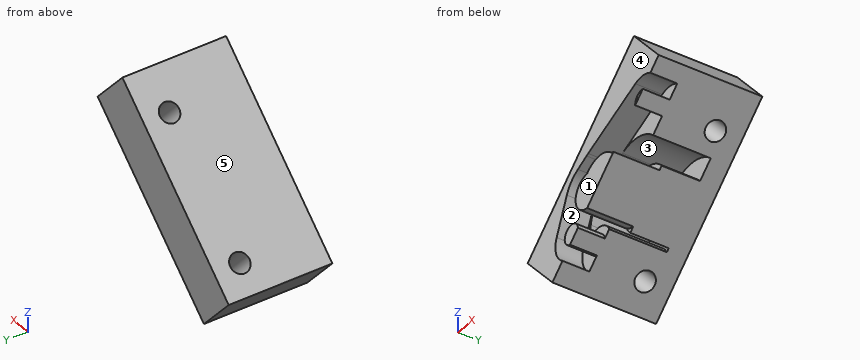
```python
from build123d import *
from build123d.topology import SkipClean

# Parameters (mm, degrees)
SKETCH2_R           = 2.5
BOSS_EXTRUDE1_DEPTH = 7
FILLET1_R           = 90
BOSS_EXTRUDE3_DEPTH = 15
SKETCH4_R           = 8
CUT_EXTRUDE1_DEPTH  = 10
BOSS_EXTRUDE4_START = 10
BOSS_EXTRUDE4_DEPTH = 10
BOSS_EXTRUDE5_DEPTH = 27
SKETCH7_R           = 2.5
CUT_EXTRUDE2_DEPTH  = 37
INTERSECT3_DEPTH    = 27


with BuildPart() as part:
    # Sketch2 → Boss-Extrude1 (new body)
    with BuildSketch(Plane(origin=(0, 0, 0), x_dir=(1, 0, 0), z_dir=(0, 1, 0))):
        with BuildLine():
            Line((-4.24846021, -9.602113613), (13.572308451, -17.486922065))
            ThreePointArc((13.572308451, -17.486922065), (20.638500285, -15.805826469), (20.907079545, -8.547382103))
            Line((20.907079545, -8.547382103), (11.451696022, 4.891208687))
            ThreePointArc((11.451696022, 4.891208687), (9.270724445, 7.034926316), (6.472222222, 8.268031175))
            ThreePointArc((6.472222222, 8.268031175), (4.86754966, 9.30359932), (3.101845071, 10.031378627))
            Line((3.101845071, 10.031378627), (-8.821699821, 13.718308443))
            ThreePointArc((-8.821699821, 13.718308443), (-15.091857172, 11.987583677), (-16.147811194, 5.569231667))
            Line((-16.147811194, 5.569231667), (-12.308520784, -3.358124948))
            ThreePointArc((-12.308520784, -3.358124948), (-9.971976629, -6.504419403), (-6.472222222, -8.268031175))
            ThreePointArc((-6.472222222, -8.268031175), (-5.401685102, -9.003987898), (-4.24846021, -9.602113613))
        make_face()
        with Locations(Location((16, -12, 0), (0, 0, 270))):
            Circle(SKETCH2_R, mode=Mode.SUBTRACT)
        with Locations(Location((-10.604337088, 7.953252816, 0), (0, 0, 270))):
            Circle(SKETCH2_R, mode=Mode.SUBTRACT)
        with BuildLine():
            ThreePointArc((-4.694444444, -4.495797077), (0, -6.5), (4.694444444, -4.495797077))
            ThreePointArc((4.694444444, -4.495797077), (9, 0), (4.694444444, 4.495797077))
            ThreePointArc((4.694444444, 4.495797077), (0, 6.5), (-4.694444444, 4.495797077))
            ThreePointArc((-4.694444444, 4.495797077), (-9, 0), (-4.694444444, -4.495797077))
        make_face(mode=Mode.SUBTRACT)
    extrude(amount=BOSS_EXTRUDE1_DEPTH)

    # Fillet1
    fillet1_edges = [part.edges().sort_by_distance(p)[0] for p in [
        (6.472222222, 3.5, -8.268031175),
        (-6.472222222, 3.5, 8.268031175),
    ]]
    fillet(fillet1_edges, radius=FILLET1_R)

    # Sketch3 → Boss-Extrude3 (add)
    with BuildSketch(Plane(origin=(0, 7, 0), x_dir=(1, 0, 0), z_dir=(0, 1, 0))):
        with BuildLine():
            Line((-13.446880098, 1.012795393), (-12.308520784, -3.358124948))
            ThreePointArc((-12.308520784, -3.358124948), (-10.611843956, -5.907229762), (-8.121968415, -7.689690813))
            ThreePointArc((-8.121968415, -7.689690813), (-6.480430757, -8.483296944), (-4.855306799, -9.309994408))
            ThreePointArc((-4.855306799, -9.309994408), (-4.554226262, -9.460920841), (-4.24846021, -9.602113613))
            Line((-4.24846021, -9.602113613), (-1.454246479, -10.838414946))
            ThreePointArc((-1.454246479, -10.838414946), (10.979115699, -7.880432641), (11.451696022, 4.891208687))
            ThreePointArc((11.451696022, 4.891208687), (9.968863726, 6.507036925), (8.121968415, 7.689690813))
            ThreePointArc((8.121968415, 7.689690813), (6.480430757, 8.483296944), (4.855306799, 9.309994408))
            ThreePointArc((4.855306799, 9.309994408), (3.994892398, 9.710346787), (3.101845071, 10.031378627))
            Line((3.101845071, 10.031378627), (-3.895223267, 11.305534387))
            ThreePointArc((-3.895223267, 11.305534387), (-5.691953988, 10.727471116), (-6.207623157, 8.911848981))
            ThreePointArc((-6.207623157, 8.911848981), (-7.30582589, 4.892236012), (-11.232333003, 3.497288147))
            ThreePointArc((-11.232333003, 3.497288147), (-13.004436636, 2.847636589), (-13.446880098, 1.012795393))
        make_face()
        with BuildLine():
            ThreePointArc((4.694444444, -4.495797077), (9, 0), (4.694444444, 4.495797077))
            ThreePointArc((4.694444444, 4.495797077), (0, 6.5), (-4.694444444, 4.495797077))
            ThreePointArc((-4.694444444, 4.495797077), (-9, 0), (-4.694444444, -4.495797077))
            ThreePointArc((-4.694444444, -4.495797077), (0, -6.5), (4.694444444, -4.495797077))
        make_face(mode=Mode.SUBTRACT)
    extrude(amount=BOSS_EXTRUDE3_DEPTH)

    # Sketch4 → Cut-Extrude1 (cut)
    with BuildSketch(Plane(origin=(0, 22, 0), x_dir=(1, 0, 0), z_dir=(0, 1, 0))):
        Circle(SKETCH4_R)
    extrude(amount=-CUT_EXTRUDE1_DEPTH, mode=Mode.SUBTRACT)

    # Sketch5 → Boss-Extrude4 (add)
    with SkipClean():  # the faces are left unmerged after this step: merging them gives an invalid solid
        with BuildSketch(Plane(origin=(0, 12, 0), x_dir=(1, 0, 0), z_dir=(0, 1, 0)).offset(BOSS_EXTRUDE4_START)):
            with BuildLine():
                ThreePointArc((-7.111111111, 3.664982778), (-8, 0), (-7.111111111, -3.664982778))
                ThreePointArc((-7.111111111, -3.664982778), (-9, 0), (-7.111111111, 3.664982778))
            make_face()
            with BuildLine():
                ThreePointArc((7.111111111, -3.664982778), (9, 0), (7.111111111, 3.664982778))
                ThreePointArc((7.111111111, 3.664982778), (8, 0), (7.111111111, -3.664982778))
            make_face()
        extrude(amount=-BOSS_EXTRUDE4_DEPTH)


with BuildPart() as body_2:
    # Sketch6 → Boss-Extrude5 (new body)
    with BuildSketch(Plane(origin=(0, 0, 0), x_dir=(-1, 0, 0), z_dir=(0, -1, 0))):
        Polygon((8.401052482, 26.937158796), (-31.729302738, -9.377746691), (-13.016359271, -30.388770935), (27.113995949, 5.926134553), align=None)
    extrude(amount=-BOSS_EXTRUDE5_DEPTH)

    # Sketch7 → Cut-Extrude2 (cut)
    with BuildSketch(Plane(origin=(-9.25873614, 0, 10.23151142), x_dir=(0.7414761288495602, 0, 0.670979247329059), z_dir=(-0.670979247329059, 0, 0.7414761288495602))):
        with Locations((-16.542969249, 20.228212297)):
            Circle(SKETCH7_R)
        with Locations((19.254983261, 20.228212297)):
            Circle(SKETCH7_R)
    extrude(amount=-CUT_EXTRUDE2_DEPTH, mode=Mode.SUBTRACT)

    # Intersect1: read off the stored shape, not the designer's step
    # Intersect1: cut part
    add(part.part, mode=Mode.SUBTRACT)

    # Intersect3: read off the stored shape, not the designer's step
    # Intersect3 outline → Intersect3 (cut)
    with BuildSketch(Plane(origin=(0, 0, 0), x_dir=(1, 0, 0), z_dir=(0, 1, 0))):
        Polygon((22.372831004, -19.883258813), (31.729302738, -9.377746691), (-8.401052482, 26.937158796), (-17.757524215, 16.431646675), align=None)
    extrude(amount=INTERSECT3_DEPTH, mode=Mode.SUBTRACT)


solid = body_2.part
```
The model under review builds one solid part; all positions refer to its coordinate system, in mm. Face numbers are marked on the shaded views. A direction names the side the tool comes from. Coordinates: 2 decimals unless noted, no trailing zeros. Write each loop counter-clockwise with the first axis right and the second up, starting at its lowest first coordinate (ties: lowest second). Pieces come first, ordered by that corner, then holes.
1) The part is to be moulded in two halves that separate along Z. For the marked faces 3, 4 and 5, say which applies: pulls with the +Z half, pulls with the -Z half, needs draft (parallel to the pull), parting line crosses it, or undercut.
2) We need section A-A on y = 15.5. State the section outline as (x, z) points, then the cut area to 3 significant figures.
3) Clearance check with flat-ended pins moving along their axes: pin 1 Ø6 at (y, z) = (21, 18) entering from -X; pin 2 Ø3 at (x, z) = (12, 13.5) entering from -Y; pin 3 Ø12 at (y, z) = (12, -10) entering from +X; pin 4 Ø12 at (x, z) = (-14, 19) entering from -Y. State where each tip first meets the part, or that it passes through.
4) To check wall thickness, follow probe 1 along Z at (x, y) = (-12.5, 2); probe 2 along Z at (x, y) = (-11, 13.5); probe 3 along X at (y, z) = (11.5, -4). State the ranges of each line that lie inside material, in increasing order.
5) We need section C-C on y = 2. Count the separate pieces of the cut face and the enclosed holes in it, then the cut area to 3 significant figures.
6) We need section B-B on y = 10.25. State the section outline as (x, z) points, then the cut area to 3 significant figures.
7) Machinability: for the marked faces 1 and 2, which of the approach directions +Z, -Z, +X, -X, +Y, -Y give a long, thin tool a straight path to every point of the face, cutting with its end or side? Answer none if there is none.
Answer list:
1. face 3: undercut
1. face 4: needs draft
1. face 5: pulls with the +Z half
2. outline: (-27.11, -5.93) - (-17.76, -16.43) - (-6.46, -6.21) arc R4.5 ccw to (-11.23, -3.5) arc R2 cw to (-13.45, -1.01) - (-12.31, 3.36) arc R8.5 cw to (-8.12, 7.69) arc R90 ccw to (-4.86, 9.31) arc R10.5 cw to (-4.25, 9.6) - (-1.45, 10.84) arc R10.56 cw to (10.13, 8.8) - (22.37, 19.88) - (13.02, 30.39) - close; (-5.75, -5.56) - (6.11, 5.17) arc R8 ccw (long way) to start
2. area: 644 mm2
3. pin 1: stops at x = -3.99
3. pin 2: stops at y = 7
3. pin 3: stops at x = -4.02
3. pin 4: passes through
4. probe 1: z = -9.58 to -6.32, 2.91 to 7.3
4. probe 2: z = -10.32 to -3.47, 5.48 to 8.66
4. probe 3: x = -24.99 to -8.45, -6.56 to -4.02
5. separate pieces: 4
5. enclosed holes: 0
5. area: 513 mm2
6. outline: (-27.11, -5.93) - (-17.76, -16.43) - (-6.46, -6.21) arc R4.5 ccw to (-11.23, -3.5) arc R2 cw to (-13.45, -1.01) - (-12.31, 3.36) arc R8.5 cw to (-8.12, 7.69) arc R90 ccw to (-4.86, 9.31) arc R10.5 cw to (-4.25, 9.6) - (-1.45, 10.84) arc R10.56 cw to (10.13, 8.8) - (22.37, 19.88) - (13.02, 30.39) - close; (-4.69, -4.5) arc R6.5 ccw to (-4.64, -4.56) - (5.3, 4.43) arc R4.5 ccw to (4.69, 4.5) arc R6.5 ccw to (-4.69, 4.5) arc R4.5 ccw to start
6. area: 628 mm2
7. face 1: +Z, -Z, +X, -X, -Y
7. face 2: -Y
